Could you check a few things on this model? Use its own coordinates, in mm. Round coordinates to 2 decimals unless told otherwise and drop trailing zeros. Loops run counter-clockwise (first coordinate to the right, second up) from the corner with the lowest first, then second, coordinate; pieces in that order, holes last. Notation, with made-up numbers: (-2, 16) - (45, 16) arc R19 cw to (45, 37) - close; hole circle Ø7 at (65, -10.75). An arc over 180 degrees is marked (long way). Answer as CSV lines item,"result". Start each with the question number.
1) Suppose I cut it at A-A, the plane z = 83. Write out the boundary of the cut face in (x, y).
2) Please list where these lines run through material, in increasing order: line 1 along Z through (x, y) = (11.5, 0.3); line 2 along X through (y, z) = (1, 0); line 3 along X through (y, z) = (1.8, 107).
3) Suppose I cut it at B-B, the plane y = 1.5. Count the separate pieces of the cut face and the enclosed holes in it, then the cut area to 3 significant figures.
4) I'm going to push flat-ended pins straight in: pin 1 Ø1.5 at (x, y) = (4, 3.5) entering from +Z; pin 2 Ø2 at (y, z) = (1.5, -115) entering from -X; pin 3 Ø3 at (y, z) = (3.5, 32) entering from +X. Where does each tip first touch, or does it pass through?
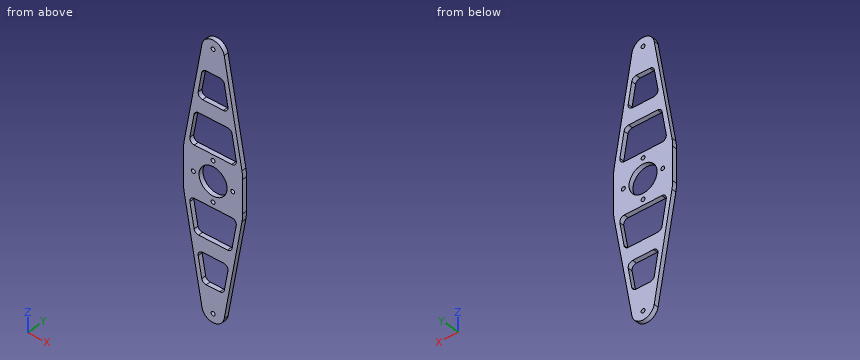
```python
from build123d import *

# Parameters (mm, degrees)
BOSS_EXTRUDE1_DEPTH     = 5
CUT_EXTRUDE1_DEPTH      = 153.164632892
CUT_EXTRUDE1_DEPTH_BACK = 153.164632892
SKETCH2_R               = 15.5
SKETCH2_R_2             = 2.15
CUT_EXTRUDE2_DEPTH      = 153.164632892
CUT_EXTRUDE2_DEPTH_BACK = 153.164632892
SKETCH3_R               = 2.2


with BuildPart() as part:
    # Sketch1 → Boss-Extrude1 (new body)
    with BuildSketch(Plane(origin=(0, 0, 0), x_dir=(1, 0, 0), z_dir=(0, 1, 0))):
        with BuildLine():
            Line((-12.310096913, 138.193763743), (-31.950416611, 26.807975707))
            ThreePointArc((-31.950416611, 26.807975707), (-32.519763865, 22.483353961), (-32.71002896, 18.125566824))
            Line((-32.71002896, 18.125566824), (-32.71002896, -18.125566824))
            ThreePointArc((-32.71002896, -18.125566824), (-32.519763865, -22.483353961), (-31.950416611, -26.807975707))
            Line((-31.950416611, -26.807975707), (-12.310096913, -138.193763743))
            ThreePointArc((-12.310096913, -138.193763743), (0, -148.523161522), (12.310096913, -138.193763743))
            Line((12.310096913, -138.193763743), (31.950416611, -26.807975707))
            ThreePointArc((31.950416611, -26.807975707), (32.519763865, -22.483353961), (32.71002896, -18.125566824))
            Line((32.71002896, -18.125566824), (32.71002896, 18.125566824))
            ThreePointArc((32.71002896, 18.125566824), (32.519763865, 22.483353961), (31.950416611, 26.807975707))
            Line((31.950416611, 26.807975707), (12.310096913, 138.193763743))
            ThreePointArc((12.310096913, 138.193763743), (0, 148.523161522), (-12.310096913, 138.193763743))
        make_face()
        with BuildLine():
            Line((12.512772117, 108.250483124), (16.422284735, 86.078535291))
            ThreePointArc((16.422284735, 86.078535291), (15.328468186, 81.996356354), (11.49824597, 80.210294402))
            Line((11.49824597, 80.210294402), (-11.49824597, 80.210294402))
            ThreePointArc((-11.49824597, 80.210294402), (-15.328468186, 81.996356354), (-16.422284735, 86.078535291))
            Line((-16.422284735, 86.078535291), (-12.512772117, 108.250483124))
            ThreePointArc((-12.512772117, 108.250483124), (-10.802671401, 111.212464452), (-7.588733352, 112.382242236))
            Line((-7.588733352, 112.382242236), (7.588733352, 112.382242236))
            ThreePointArc((7.588733352, 112.382242236), (10.802671401, 111.212464452), (12.512772117, 108.250483124))
        make_face(mode=Mode.SUBTRACT)
        with BuildLine():
            Line((-16.065250357, 64.309525453), (16.065250357, 64.309525453))
            ThreePointArc((16.065250357, 64.309525453), (19.279188405, 63.139747668), (20.989289122, 60.177766341))
            Line((20.989289122, 60.177766341), (25.626657813, 33.877941591))
            ThreePointArc((25.626657813, 33.877941591), (24.532841264, 29.795762655), (20.702619048, 28.009700703))
            Line((20.702619048, 28.009700703), (-20.702619048, 28.009700703))
            ThreePointArc((-20.702619048, 28.009700703), (-24.532841264, 29.795762655), (-25.626657813, 33.877941591))
            Line((-25.626657813, 33.877941591), (-20.989289122, 60.177766341))
            ThreePointArc((-20.989289122, 60.177766341), (-19.279188405, 63.139747668), (-16.065250357, 64.309525453))
        make_face(mode=Mode.SUBTRACT)
        with BuildLine():
            Line((-7.588733352, -112.382242236), (7.588733352, -112.382242236))
            ThreePointArc((7.588733352, -112.382242236), (10.802671401, -111.212464452), (12.512772117, -108.250483124))
            Line((12.512772117, -108.250483124), (16.422284735, -86.078535291))
            ThreePointArc((16.422284735, -86.078535291), (15.328468186, -81.996356354), (11.49824597, -80.210294402))
            Line((11.49824597, -80.210294402), (-11.49824597, -80.210294402))
            ThreePointArc((-11.49824597, -80.210294402), (-15.328468186, -81.996356354), (-16.422284735, -86.078535291))
            Line((-16.422284735, -86.078535291), (-12.512772117, -108.250483124))
            ThreePointArc((-12.512772117, -108.250483124), (-10.802671401, -111.212464452), (-7.588733352, -112.382242236))
        make_face(mode=Mode.SUBTRACT)
        with BuildLine():
            Line((-20.989289122, -60.177766341), (-25.626657813, -33.877941591))
            ThreePointArc((-25.626657813, -33.877941591), (-24.532841264, -29.795762655), (-20.702619048, -28.009700703))
            Line((-20.702619048, -28.009700703), (20.702619048, -28.009700703))
            ThreePointArc((20.702619048, -28.009700703), (24.532841264, -29.795762655), (25.626657813, -33.877941591))
            Line((25.626657813, -33.877941591), (20.989289122, -60.177766341))
            ThreePointArc((20.989289122, -60.177766341), (19.279188405, -63.139747668), (16.065250357, -64.309525453))
            Line((16.065250357, -64.309525453), (-16.065250357, -64.309525453))
            ThreePointArc((-16.065250357, -64.309525453), (-19.279188405, -63.139747668), (-20.989289122, -60.177766341))
        make_face(mode=Mode.SUBTRACT)
    extrude(amount=BOSS_EXTRUDE1_DEPTH)

    # Sketch2 → Cut-Extrude1 (cut, two sides: drawn at the far end of the back side and taken through both)
    with BuildSketch(Plane(origin=(0, 5, 0), x_dir=(1, 0, 0), z_dir=(0, 1, 0)).offset(-CUT_EXTRUDE1_DEPTH_BACK)):
        with Locations(Location((0, 0, 0), (0, 0, 270))):
            Circle(SKETCH2_R)
        with Locations(Location((0, 21.754850352, 0), (0, 0, 270))):
            Circle(SKETCH2_R_2)
        with Locations(Location((21.754850352, 0, 0), (0, 0, 270))):
            Circle(SKETCH2_R_2)
        with Locations(Location((0, -21.754850352, 0), (0, 0, 270))):
            Circle(SKETCH2_R_2)
        with Locations(Location((-21.754850352, 0, 0), (0, 0, 270))):
            Circle(SKETCH2_R_2)
    extrude(amount=CUT_EXTRUDE1_DEPTH + CUT_EXTRUDE1_DEPTH_BACK, mode=Mode.SUBTRACT)

    # Sketch3 → Cut-Extrude2 (cut, two sides: drawn at the far end of the back side and taken through both)
    with BuildSketch(Plane.XZ.offset(-CUT_EXTRUDE2_DEPTH_BACK)):
        with Locations(Location((0, -139, 0), (0, 0, 270))):
            Circle(SKETCH3_R)
        with Locations(Location((0, 139, 0), (0, 0, 270))):
            Circle(SKETCH3_R)
    extrude(amount=CUT_EXTRUDE2_DEPTH + CUT_EXTRUDE2_DEPTH_BACK, mode=Mode.SUBTRACT)


solid = part.part
```
Filled sheet:
1,outline,"(-22.04, 0) - (-15.98, 0) - (-15.98, 5) - (-22.04, 5) - close; (15.98, 0) - (22.04, 0) - (22.04, 5) - (15.98, 5) - close"
2,line 1,"-140.92 to -110.5, -80.21 to -64.31, -28.01 to -10.39, 10.39 to 28.01, 64.31 to 80.21, 110.5 to 140.92"
2,line 2,"-32.71 to -23.9, -19.6 to -15.5, 15.5 to 19.6, 23.9 to 32.71"
2,line 3,"-17.81 to -12.73, 12.73 to 17.81"
3,separate pieces,"1"
3,enclosed holes,"11"
3,area,"7,700 mm²"
4,pin 1,"z = 148.09"
4,pin 2,"x = -16.58"
4,pin 3,"x = 31.3"
